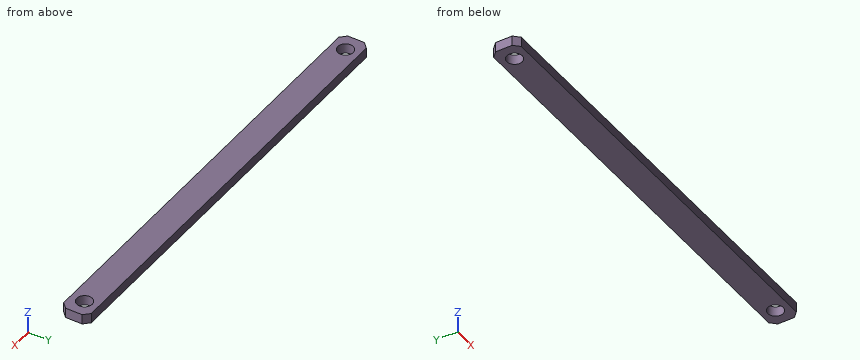
```python
from build123d import *

# Parameters (mm, degrees)
SKETCH_1_R      = 7
EXTRUDE_1_DEPTH = 4.5


with BuildPart() as part:
    # 草圖1 → 填料-伸長1 (new body, symmetric)
    with BuildSketch(Plane.XY):
        Polygon((195, 12.5), (200, 7.5), (200, -7.5), (195, -12.5), (-195, -12.5), (-200, -7.5), (-200, 7.5), (-195, 12.5), align=None)
        with Locations((185, 0)):
            Circle(SKETCH_1_R, mode=Mode.SUBTRACT)
        with Locations((-185, 0)):
            Circle(SKETCH_1_R, mode=Mode.SUBTRACT)
    extrude(amount=EXTRUDE_1_DEPTH, both=True)


solid = part.part
```
Verification items for the finished model (mm, model axes). Coordinates: 2 decimals unless noted, no trailing zeros. Order: outer loops, then holes, each group sorted by start corner. A loop starts at its lowest first (then second) coordinate and runs counter-clockwise, first axis right, second up. Notation, with made-up numbers: (77, -26) -> (115, -26) arc R21 cw to (115, -18) -> close; hole circle Ø7 at (14.5, 11.25). An arc over 180 degrees is marked (long way). Put each result on its own line as item: value. Start each with the question number.
1) Cross-section at C-C (x = 185). Enter the section's corners in (y, z), plus the area to 3 significant figures.
2) Material ranges on L1, parallel to X at y = 1, z = -3; L2, parallel to Y at x = 185, z = 2.25; L3, parallel to X at y = 4.5, z = 1.5, recorded low to high.
3) Cross-section at B-B (z = -2.75). Enter the section's corners in (x, y), plus the area to 3 significant figures.
4) Cross-section at A-A (y = 0). Enter the section's corners in (x, z).
Geometry check:
1. outline: (-12.5, -4.5) -> (-7, -4.5) -> (-7, 4.5) -> (-12.5, 4.5) -> close; (7, -4.5) -> (12.5, -4.5) -> (12.5, 4.5) -> (7, 4.5) -> close
1. area: 99.0 mm^2
2. L1: x = -200 to -191.93, -178.07 to 178.07, 191.93 to 200
2. L2: y = -12.5 to -7, 7 to 12.5
2. L3: x = -200 to -190.36, -179.64 to 179.64, 190.36 to 200
3. outline: (-200, -7.5) -> (-195, -12.5) -> (195, -12.5) -> (200, -7.5) -> (200, 7.5) -> (195, 12.5) -> (-195, 12.5) -> (-200, 7.5) -> close; hole circle Ø14 at (-185, 0); hole circle Ø14 at (185, 0)
3. area: 9,640 mm^2
4. outline: (-200, -4.5) -> (-192, -4.5) -> (-192, 4.5) -> (-200, 4.5) -> close; (-178, -4.5) -> (178, -4.5) -> (178, 4.5) -> (-178, 4.5) -> close; (192, -4.5) -> (200, -4.5) -> (200, 4.5) -> (192, 4.5) -> close
